The model under review builds one solid part; all positions refer to its coordinate system, in mm. Face numbers are marked on the shaded views. A direction names the side the tool comes from. Give positions to 0.01 mm unless a question says otherwise; leave off trailing zeros. Write each loop counter-clockwise with the first axis right and the second up, starting at its lowest first coordinate (ties: lowest second). Pieces come first, ordered by that corner, then holes. Notation, with made-up numbers: M 21,55.25 L 54,55.25 A15 cw 54,79.25 Z; hole C 48,77 d5. An arc over 180 degrees is marked long. Write each question's results on one line, items separated by ' | '. Start each with the question number.
from build123d import *

# Parameters (mm, degrees)
SKETCH_1_W      = 40
SKETCH_1_H      = 6
SKETCH_1_R      = 1.75
EXTRUDE_1_DEPTH = 3.75
SKETCH_2_W      = 6
SKETCH_2_H      = 9.75
EXTRUDE_2_DEPTH = 32


with BuildPart() as part:
    # 草图1 → 凸台-拉伸1 (new body)
    with BuildSketch(Plane(origin=(0, 0, 0), x_dir=(1, 0, 0), z_dir=(0, 1, 0))):
        Rectangle(SKETCH_1_W, SKETCH_1_H)
        with Locations(Location((-15, 0, 0), (0, 0, 270))):
            Circle(SKETCH_1_R, mode=Mode.SUBTRACT)
        with Locations(Location((5, 0, 0), (0, 0, 270))):
            Circle(SKETCH_1_R, mode=Mode.SUBTRACT)
    extrude(amount=EXTRUDE_1_DEPTH)

    # 草图2 → 凸台-拉伸2 (add)
    with BuildSketch(Plane(origin=(20, 0, 0), x_dir=(0, 0, -1), z_dir=(1, 0, 0))):
        with Locations((0, -1.125)):
            Rectangle(SKETCH_2_W, SKETCH_2_H)
    extrude(amount=EXTRUDE_2_DEPTH)


solid = part.part
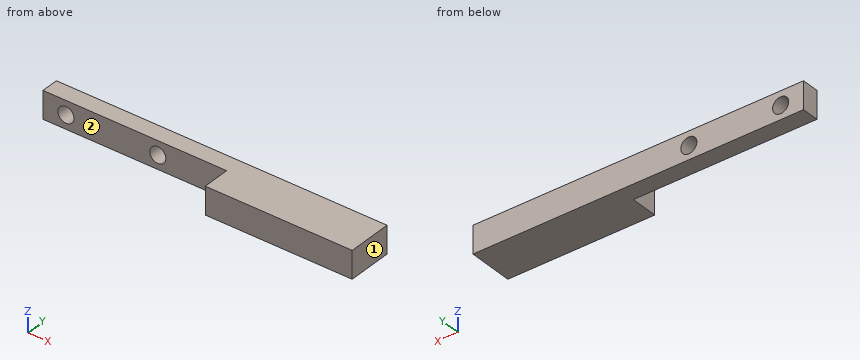
(1) Add section B-B (z = 0). State the section outline as (x, y) points, then the cut area to 3 significant figures.
(2) Clearance check with flat-ended pins moving along their axes: P1, Ø3, axis at y = -4, z = -1, coming from the -X side; P2, Ø1.8, axis at x = -9.5, z = 0.5, coming from the -Y side. State where each tip first meets the part, or that it passes through.
(3) Add section A-A (x = -15). State the section outline as (y, z) points, then the cut area to 4 significant figures.
(4) Machinability: for the marked faces 1 and 2, which of the approach directions +Z, -Z, +X, -X, +Y, -Y give a long, thin tool a straight path to every point of the face, cutting with its end or side? Answer none if there is none.
(5) Add section C-C (y = 1.5). State the section outline as (x, z) points.
(6) Wall thickness on L1, parallel to X at y = 0.95, z = 0; L2, parallel to X at y = 1.5, z = 0.7; L3, parallel to Y at x = -13.5, z = -1.35: over which ranges is each line inside the solid? List them lowest first.
(7) Add section D-D (y = -1.75). State the section outline as (x, z) points.
Calculated:
1) outline: M -20,0 L -16.75,0 L -16.75,3.75 L -20,3.75 Z; M -13.25,0 L 3.25,0 L 3.25,3.75 L -13.25,3.75 Z; M 6.75,0 L 20,0 L 20,-6 L 52,-6 L 52,3.75 L 6.75,3.75 Z | area: 436 mm²
2) P1: stops at x = 20 | P2: stops at y = 0
3) outline: M 0,-3 L 3.75,-3 L 3.75,-1.75 L 0,-1.75 Z; M 0,1.75 L 3.75,1.75 L 3.75,3 L 0,3 Z | area: 9.375 mm²
4) face 1: +Z, -Z, +X, +Y, -Y | face 2: +Z, -Z, -X, -Y
5) outline: M -20,-3 L 52,-3 L 52,3 L -20,3 Z; hole C -15,0 d3.5; hole C 5,0 d3.5
6) L1: x = -20 to -16.75, -13.25 to 3.25, 6.75 to 52 | L2: x = -20 to -16.6, -13.4 to 3.4, 6.6 to 52 | L3: y = 0 to 3.75
7) outline: M 20,-3 L 52,-3 L 52,3 L 20,3 Z
